Part model, mm, in its own coordinate system. Face numbers are marked on the shaded views. A direction names the side the tool comes from. Round coordinates to 2 decimals unless told otherwise and drop trailing zeros. Write each loop counter-clockwise with the first axis right and the second up, starting at its lowest first coordinate (ties: lowest second). Pieces come first, ordered by that corner, then holes.
1) Drill centre lines: L1, parallel to X at y = 0, z = 5; L2, parallel to Y at x = -17.75, z = 3.75; L3, parallel to Y at x = -15.5, z = 8.75. Where is each one in solid material? Low to high.
2) Saw through at D-D on y = -5.5. Write the cut outline in (x, z).
3) Saw through at A-A on x = 0. Write the cut outline in (y, z).
4) Which spindle directions (+Z, -Z, +X, -X, +Y, -Y) get a long thin tool onto all of the face, cutting with end or side? Do the marked faces 1, 2 and 3. Say none if no direction does.
5) Pull direction Y, two halves, no side cores. Call the marked faces 4, 5 and 6: +Y half, -Y half, draft (parallel to the pull), parting line (faces both ways), or undercut.
6) Flat gauge pins, fed straight in: pin 1 (4 mm diameter, centred on x = -12, z = 1.5, fed in from -Y); pin 2 (6 mm diameter, centred on y = 0.5, z = 1.5, fed in from +X); pin 3 (2 mm diameter, centred on y = 1, z = 8.5, fed in from -X); pin 4 (4 mm diameter, centred on x = -17, z = 2, fed in from +Y). Where does each tip first touch, or does it go through?
7) Saw through at C-C on z = 4.75. Write the cut outline in (x, y), and give its area (3 significant figures).
8) Saw through at B-B on y = 4. Write the cut outline in (x, z).
Autodesk Inventor part; units mm, degrees
ref_plane "YZ Plane" through (0, 0, 0) normal (1, 0, 0) x (0, 1, 0)
ref_plane "XZ Plane" through (0, 0, 0) normal (0, 1, 0) x (-1, 0, 0)
ref_plane "XY Plane" through (0, 0, 0) normal (0, 0, 1) x (1, 0, 0)
sketch "Sketch1" plane through (0, 0, 0) normal (0, 0, 1) x (1, 0, 0)
  circle A0 centre (0, 0) radius 2.5
  circle A1 centre (0, 0) radius 5
  line L0 (-1.7678, -1.7678) -> (-12.3744, 8.8388)
  line L1 (-12.3744, 8.8388) -> (-15.9099, 5.3033)
  line L2 (-15.9099, 5.3033) -> (-15.9099, 0.3033)
  line L3 (-15.9099, 0.3033) -> (1.7678, -17.3744)
  line L4 (1.7678, -17.3744) -> (1.7678, -26.5165)
  line L5 (1.7678, -26.5165) -> (-6.7678, -35.052)
  line L6 (-6.7678, -35.052) -> (-20.9099, -20.9099)
  line L7 (1.7678, 1.7678) -> (-12.3744, 15.9099)
  line L8 (-12.3744, 15.9099) -> (-20.9099, 7.3744)
  line L9 (-20.9099, 7.3744) -> (-20.9099, -1.7678)
  line L10 (-20.9099, -1.7678) -> (-3.2322, -19.4454)
  line L11 (-3.2322, -19.4454) -> (-3.2322, -24.4454)
  line L12 (-3.2322, -24.4454) -> (-6.7678, -27.981)
  line L13 (-6.7678, -27.981) -> (-17.3744, -17.3744)
  line L14 (-17.3744, -17.3744) -> (-20.9099, -20.9099)
  line L15 (-1.7678, -1.7678) -> (1.7678, 1.7678)
  circle A2 centre (-19.1421, -19.1421) radius 2.5
  circle A3 centre (-19.1421, -19.1421) radius 5
  dimension "d0" = 5
  dimension "d1" = 10
  dimension "d3" = 90
  dimension "d4" = 135
  dimension "d5" = 135
  dimension "d6" = 135
  dimension "d7" = 135
  dimension "d8" = 90
  dimension "d9" = 5
  dimension "d12" = 10
  dimension "d13" = 15
  dimension "d14" = 15
  dimension "d15" = 5
  dimension "d16" = 5
  dimension "d17" = 5
  dimension "d18" = 5
  dimension "d20" = 20
  dimension "d21" = 20
  dimension "d22" = 5
  dimension "d23" = 5
  dimension "d24" = 5
extrude "Extrusion2" add sketch "Sketch1" along normal blind 10 contours A0 L7 A1 L0 | A0 L0 A1 L7 | A1 L0 L1 L2 L3 L4 L5 L6 A3 L13 L12 L11 L10 L9 L8 L7 | A3 L6 A2 L13 | L13 A2 L6 A3 | A2 L14 picked at (-18.68, -20.1685)
sketch "Sketch2" plane through (0, 0, 10) normal (0, 0, 1) x (1, 0, 0)
  line L0 (-1.2941, 4.8296) -> (-12.3744, 15.9099)
  line L1 (-12.3744, 15.9099) -> (-20.9099, 7.3744)
  line L2 (-20.9099, 7.3744) -> (-20.9099, -1.7678)
  line L3 (-20.9099, -1.7678) -> (-3.2322, -19.4454)
  line L4 (-3.2322, -19.4454) -> (-3.2322, -24.4454)
  line L5 (-3.2322, -24.4454) -> (-6.7678, -27.981)
  line L6 (-6.7678, -27.981) -> (-14.3125, -20.4362)
  arc A0 (-14.3125, -20.4362) -> (-17.848, -23.9718) centre (-19.1421, -19.1421) ccw
  line L7 (-17.848, -23.9718) -> (-6.7678, -35.052)
  line L8 (-6.7678, -35.052) -> (1.7678, -26.5165)
  line L9 (1.7678, -26.5165) -> (1.7678, -17.3744)
  line L10 (1.7678, -17.3744) -> (-15.9099, 0.3033)
  line L11 (-15.9099, 0.3033) -> (-15.9099, 5.3033)
  line L12 (-15.9099, 5.3033) -> (-12.3744, 8.8388)
  line L13 (-12.3744, 8.8388) -> (-4.8296, 1.2941)
  arc A1 (-4.8296, 1.2941) -> (-1.2941, 4.8296) centre (0, 0) ccw
  line L14 (-20.9099, -20.9099) -> (-17.3744, -17.3744)
  arc A2 (-17.3744, -17.3744) -> (-20.9099, -20.9099) centre (-19.1421, -19.1421) ccw
  circle A3 centre (0, 0) radius 2.5
  circle A4 centre (-19.1421, -19.1421) radius 2.5
extrude "Extrusion3" cut sketch "Sketch2" against normal blind 10 contours L14 A4
equation "\"d1\" = 2 * d0"
equation "\"d9\" = d0"
equation "\"d12\" = d1"
equation "\"d13\" = 3 * d0"
equation "\"d14\" = d13"
equation "\"d15\" = d0"
equation "\"d17\" = d15"
equation "\"d18\" = d16"
properties part number "Sawaiz Logo"
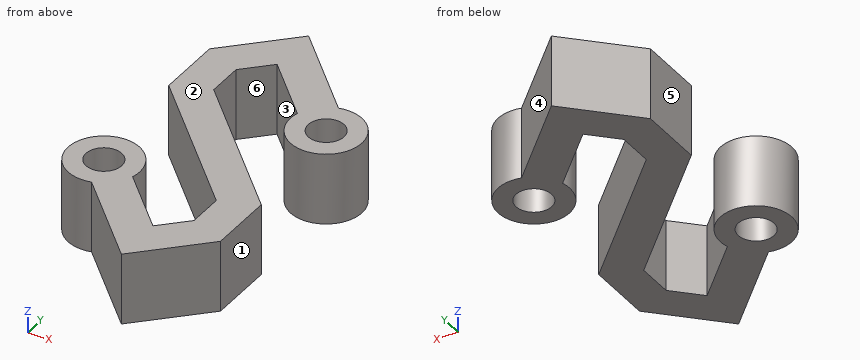
Completed:
1. L1: x = -20.91 to -15.61, -5 to -2.5, 2.5 to 5
1. L2: y = -24.07 to -21.22, -17.07 to -14.34, -4.93 to 10.53
1. L3: y = -26.32 to -15.72, -7.18 to -0.11, 5.71 to 12.78
2. outline: (-17.18, 0) - (-10.11, 0) - (-10.11, 10) - (-17.18, 10) - close
3. outline: (-28.28, 0) - (-15.61, 0) - (-15.61, 10) - (-28.28, 10) - close; (-5, 0) - (-2.5, 0) - (-2.5, 10) - (-5, 10) - close; (2.5, 0) - (5, 0) - (5, 10) - (2.5, 10) - close
4. face 1: +Z, -Z, +X, -Y
4. face 2: +Z, +X, -X, +Y, -Y
4. face 3: +Z, -Z
5. face 4: +Y half
5. face 5: draft
5. face 6: undercut
6. pin 1: stops at y = -31.82
6. pin 2: stops at x = 5
6. pin 3: stops at x = -20.91
6. pin 4: stops at y = 13.28
7. outline: (-20.91, -1.77) - (-3.23, -19.45) - (-3.23, -24.45) - (-6.77, -27.98) - (-14.31, -20.44) arc R5 ccw (long way) to (-17.85, -23.97) - (-6.77, -35.05) - (1.77, -26.52) - (1.77, -17.37) - (-15.91, 0.3) - (-15.91, 5.3) - (-12.37, 8.84) - (-4.83, 1.29) arc R5 ccw (long way) to (-1.29, 4.83) - (-12.37, 15.91) - (-20.91, 7.37) - close; hole circle Ø5 at (-19.14, -19.14); hole circle Ø5 at (0, 0)
7. area: 526 mm2
8. outline: (-20.91, 0) - (-15.91, 0) - (-15.91, 10) - (-20.91, 10) - close; (-7.54, 0) - (3, 0) - (3, 10) - (-7.54, 10) - close
